from build123d import *

# Parameters (mm, degrees)
BOSS_EXTRUDE1_DEPTH = 3
SKETCH2_W           = 11.1125
SKETCH2_H           = 3
CUT_EXTRUDE1_DEPTH  = 4


with BuildPart() as part:
    # Sketch1 → Boss-Extrude1 (new body)
    with BuildSketch(Plane(origin=(0, 0, 0), x_dir=(1, 0, 0), z_dir=(0, 1, 0))):
        Polygon((-22.225, -11.5), (22.225, -11.5), (22.225, -9), (26.625, -9), (26.625, -4), (22.225, -4), (22.225, 2.5), (26.625, 2.5), (26.625, 7.5), (22.225, 7.5), (22.225, 11.5), (-22.225, 11.5), (-22.225, 7.5), (-26.625, 7.5), (-26.625, 2.5), (-22.225, 2.5), (-22.225, -4), (-26.625, -4), (-26.625, -9), (-22.225, -9), align=None)
    extrude(amount=BOSS_EXTRUDE1_DEPTH)

    # Sketch2 → Cut-Extrude1 (cut, through all)
    with BuildSketch(Plane(origin=(0, 3, 0), x_dir=(1, 0, 0), z_dir=(0, 1, 0))):
        with Locations((-16.66875, 10)):
            Rectangle(SKETCH2_W, SKETCH2_H)
        with Locations((5.55625, 10)):
            Rectangle(SKETCH2_W, SKETCH2_H)
    extrude(amount=-CUT_EXTRUDE1_DEPTH, mode=Mode.SUBTRACT)


solid = part.part
Work out the finished part from the listing and answer in its coordinate system (mm). A direction names the side the tool comes from. Give positions to 0.01 mm unless a question says otherwise; leave off trailing zeros. Order: outer loops, then holes, each group sorted by start corner. A loop starts at its lowest first (then second) coordinate and runs counter-clockwise, first axis right, second up. Notation, with made-up numbers: (55.25, -38) -> (67.25, -38) arc R24 cw to (67.25, -18) -> close; hole circle Ø1 at (24, 50). An arc over 180 degrees is marked (long way). Answer as a JSON object with one key per item and string values. Group by question number.
1. Section C-C on y = 2.5 is taken. Determine the outline of the cut face in (x, z) (1 decimal), plus the area to 3 significant figures.
2. Section A-A on x = -23 is taken. Determine the outline of the cut face in (y, z), plus the area to 3 significant figures.
3. Section D-D on z = -1.5 is taken. Determine the outline of the cut face in (x, y) (3 decimals), plus the area to 3 significant figures.
4. Section B-B on z = -9 is taken. Determine the outline of the cut face in (x, y) (1 decimal).
5. The mould has two halves that part along Z. Classify faces 4 (the flat face through (26.625, 1, 7)), 5 (the flat face through (17, 1, -11.5)), 6 (the flat face through (24, 1, 4)): released by +Z, released by -Z, zero draft, split by the parting line, or undercut.
6. Flat-ended cylindrical pins translate along their axes: pin 1 Ø0.5 at (y, z) = (1.5, -8) entering from -X (3 decimals); pin 2 Ø0.9 at (y, z) = (2, -9.5) entering from +X (3 decimals); pin 3 Ø1.5 at (y, z) = (2, -10.5) entering from -X. Find the tip coordinate at first contact, or state that the pin passes through.
7. Consider line 1 along X through (y, z) = (2.6, -9) (1 decimal); line 2 along X through (y, z) = (1.6, -7.75) (3 decimals); line 3 along Z through (x, y) = (-11.5, 1.5). Determine where each line is inside the solid, lowest interval first. Write a range as [from, to].
8. A tool of negligible diameter and unlimited length cuts with its end or side. For faces 1 (the flat face through (-24, 1, 9)), 2 (the flat face through (24, 1, -2.5)), 3 (the flat face through (-11.112, 2, -10)), from which of +Z, -Z, +X, -X, +Y, -Y can it reach the whole face along a straight path? Write none if from no direction.
Result sheet:
{
 "1": {"outline": "(-26.6, -7.5) -> (-22.2, -7.5) -> (-22.2, -8.5) -> (-11.1, -8.5) -> (-11.1, -11.5) -> (0, -11.5) -> (0, -8.5) -> (11.1, -8.5) -> (11.1, -11.5) -> (22.2, -11.5) -> (22.2, -7.5) -> (26.6, -7.5) -> (26.6, -2.5) -> (22.2, -2.5) -> (22.2, 4) -> (26.6, 4) -> (26.6, 9) -> (22.2, 9) -> (22.2, 11.5) -> (-22.2, 11.5) -> (-22.2, 9) -> (-26.6, 9) -> (-26.6, 4) -> (-22.2, 4) -> (-22.2, -2.5) -> (-26.6, -2.5) -> close", "area": "1,040 mm^2"},
 "2": {"outline": "(0, -7.5) -> (3, -7.5) -> (3, -2.5) -> (0, -2.5) -> close; (0, 4) -> (3, 4) -> (3, 9) -> (0, 9) -> close", "area": "30.0 mm^2"},
 "3": {"outline": "(-22.225, 0) -> (22.225, 0) -> (22.225, 3) -> (-22.225, 3) -> close", "area": "133 mm^2"},
 "4": {"outline": "(-11.1, 0) -> (0, 0) -> (0, 3) -> (-11.1, 3) -> close; (11.1, 0) -> (22.2, 0) -> (22.2, 3) -> (11.1, 3) -> close"},
 "5": {"face 4": "zero draft", "face 5": "released by -Z", "face 6": "undercut"},
 "6": {"pin 1": "stops at x = -22.225", "pin 2": "stops at x = 22.225", "pin 3": "stops at x = -11.11"},
 "7": {"line 1": "x = [-11.1, 0], [11.1, 22.2]", "line 2": "x = [-22.225, 22.225]", "line 3": "z = [-8.5, 11.5]"},
 "8": {"face 1": "+Z, -X, +Y, -Y", "face 2": "+X, +Y, -Y", "face 3": "-Z, -X, +Y, -Y"}
}
